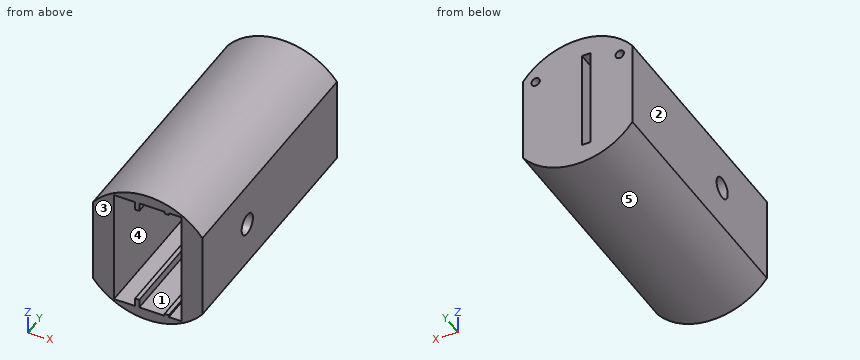
from build123d import *

# Parameters (mm, degrees)
F1_DEPTH  = 120
F2_DEPTH  = 10
F3_DEPTH  = 45
F4_D      = 4
F4_DEPTH  = 15
F4_TIP    = 1.2017212381
F6_D      = 10
F7_DEPTH  = 15
F8_W      = 2
F8_H      = 1
F9_DEPTH  = 110
F10_DEPTH = 2


with BuildPart() as f1:
    # F0 (on Front) → F1 (new body)
    with BuildSketch(Plane.XZ):
        with BuildLine():
            Line((26, -20.3224014329), (26, 20.3224014329))
            ThreePointArc((26, 20.3224014329), (0, 33), (-26, 20.3224014329))
            Line((-26, 20.3224014329), (-26, -20.3224014329))
            ThreePointArc((-26, -20.3224014329), (0, -33), (26, -20.3224014329))
        make_face()
        Polygon((-16, -27.75), (-16, 27.75), (-6, 27.75), (-6, 23.75), (-4, 23.75), (-4, 27.75), (16, 27.75), (16, -27.75), (-4, -27.75), (-4, -23.75), (-6, -23.75), (-6, -27.75), align=None, mode=Mode.SUBTRACT)
    extrude(amount=F1_DEPTH)

    # F0 (on Front) → F2 (join)
    with BuildSketch(Plane.XZ):
        Polygon((-4, 27.75), (-4, 23.75), (-4, -23.75), (-4, -27.75), (16, -27.75), (16, 27.75), align=None)
    extrude(amount=F2_DEPTH)

    # F0 (on Front) → F3 (join)
    with BuildSketch(Plane.XZ):
        Polygon((-6, 27.75), (-16, 27.75), (-16, -27.75), (-6, -27.75), (-6, -23.75), (-6, 23.75), align=None)
    extrude(amount=F3_DEPTH)

    # F4
    with Locations(Plane(origin=(0, 0, 0), x_dir=(1, 0, 0), z_dir=(0, 1, 0))):
        with Locations((20, -18), (-20, -18)):
            Hole(F4_D / 2, depth=F4_DEPTH)
            with Locations((0, 0, -(F4_DEPTH + F4_TIP / 2))):  # 118° drill point
                Cone(0, F4_D / 2, F4_TIP, mode=Mode.SUBTRACT)

    # F6 (through all)
    with Locations(Plane.YZ.offset(26)):
        with Locations((-80, 0)):
            Hole(F6_D / 2)

    # F7 (cut): a face of the model
    f7_faces = [f1.faces().sort_by_distance(p)[0] for p in [
        (-11, -45, 0),
    ]]
    extrude(f7_faces, amount=-F7_DEPTH, mode=Mode.SUBTRACT)

    # F8 (on face) → F9 (join, through all)
    with BuildSketch(Plane.XZ.offset(120)):
        with Locations((9, 27.25)):
            Rectangle(F8_W, F8_H)
        with Locations((9, -27.25)):
            Rectangle(F8_W, F8_H)
    extrude(amount=-F9_DEPTH)

    # F10 (cut): a face of the model
    f10_faces = [f1.faces().sort_by_distance(p)[0] for p in [
        (-4, -5, 0),
    ]]
    extrude(f10_faces, amount=-F10_DEPTH, mode=Mode.SUBTRACT)


solid = f1.part
Geometry: final body of the model. Coordinates: model frame, mm. Face numbers are marked on the shaded views. A direction names the side the tool comes from. Coordinates: 2 decimals unless noted, no trailing zeros. Order: outer loops, then holes, each group sorted by start corner. A loop starts at its lowest first (then second) coordinate and runs counter-clockwise, first axis right, second up. Notation, with made-up numbers: (-12, -35) - (30, -35) arc R30 ccw to (30, -6) - close; hole circle Ø1 at (83.5, 85.25). An arc over 180 degrees is marked (long way). Use one line per item in the form item = value.
1) Ray query, L1, parallel to X at y = -9.75, z = 18; L2, parallel to X at y = -72, z = -19; L3, parallel to X at y = -15, z = -10. Return the intervals inside material, ascending.
Solutions:
L1 = -26 to -22, -18 to -6, -2 to 18, 22 to 26
L2 = -26 to -16, 16 to 26
L3 = -26 to -6, 16 to 26
2) Set-up query: the marked faces 1 and 2. Return all of +Z, -Z, +X, -X, +Y, -Y with unobstructed straight access to the full face (end or side cutting, diameter ignored); none if empty.
Solutions:
face_1 = -Y
face_2 = +Z, -Z, -X, +Y, -Y
3) Section B-B (z = 0). Return loops of the section in (x, y), then the cut area to 3 significant figures.
Solutions:
outline = (-26, -120) - (-16, -120) - (-16, -85) - (-26, -85) - close; (-26, -75) - (-16, -75) - (-16, -30) - (-6, -30) - (-6, 0) - (-26, 0) - close; (-2, -10) - (16, -10) - (16, -75) - (26, -75) - (26, 0) - (-2, 0) - close; (16, -120) - (26, -120) - (26, -85) - (16, -85) - close
area = 2,680 mm^2
4) Pin query (flat end, axial travel): pin 1 (1.2 mm diameter, centred on y = -82.5, z = 26, fed in from +X); pin 2 (4.5 mm diameter, centred on x = -3, y = -36.5, fed in from +Z); pin 3 (2 mm diameter, centred on x = 4, z = -11, fed in from -Y). Return the tip coordinate at first contact, or that it passes through.
Solutions:
pin_1 = 21.07
pin_2 = 32.99
pin_3 = -10
5) Mould query, pull axis Z, two halves, no side actions, for the marked faces 3, 4 and 5. Classes: +Z half, -Z half, draft (parallel to the pull), parting line (faces both ways), or undercut.
Solutions:
face_3 = draft
face_4 = undercut
face_5 = -Z half
6) Section C-C (y = -91). Return loops of the section in (x, z).
Solutions:
outline = (-26, -20.32) arc R33 ccw to (26, -20.32) - (26, 20.32) arc R33 ccw to (-26, 20.32) - close; hole (-16, -27.75) - (-6, -27.75) - (-6, -23.75) - (-4, -23.75) - (-4, -27.75) - (8, -27.75) - (8, -26.75) - (10, -26.75) - (10, -27.75) - (16, -27.75) - (16, 27.75) - (10, 27.75) - (10, 26.75) - (8, 26.75) - (8, 27.75) - (-4, 27.75) - (-4, 23.75) - (-6, 23.75) - (-6, 27.75) - (-16, 27.75) - close
7) Section A-A (z = -8.5). Return loops of the section in (x, y).
Solutions:
outline = (-26, -120) - (-16, -120) - (-16, -30) - (-6, -30) - (-6, 0) - (-26, 0) - close; (-2, -10) - (16, -10) - (16, -120) - (26, -120) - (26, 0) - (-2, 0) - close
8) Section D-D (x = 0). Return loops of the section in (y, z).
Solutions:
outline = (-120, -33) - (0, -33) - (0, 33) - (-120, 33) - (-120, 27.75) - (-10, 27.75) - (-10, -27.75) - (-120, -27.75) - close
